Source: CAD feature listing. Evaluate the final solid. Frame: model axes, mm. A direction names the side the tool comes from. Round coordinates to 2 decimals unless told otherwise and drop trailing zeros. Loops run counter-clockwise (first coordinate to the right, second up) from the corner with the lowest first, then second, coordinate; pieces in that order, holes last. Notation, with made-up numbers: (50.25, 37) -> (100.25, 37) arc R33 ccw to (100.25, 73) -> close; hole circle Ø6 at (2, 25.5). An arc over 180 degrees is marked (long way). Put each result on its own line as item: value. Start each with the question number.
1. Contact query for flat-ended pins moving along their axis: pin 1 (6.5 mm diameter, centred on x = -65, y = 8, fed in from +Z); pin 2 (4.5 mm diameter, centred on y = 7, z = -56.5, fed in from +X); pin 3 (4 mm diameter, centred on x = -5.5, y = 10.5, fed in from -Z). Output: stop coordinate, or through.
2. Cut plane B-B (x = -39). Return the cut outline in (y, z), then the cut area to 3 significant figures.
3. Set-up query: faces 5 (the flat face through (49, 9, 56)), 6 (the flat face through (-13, 9, 56)), 7 (the flat face through (-17.1, 7.8, 54.25)). Return all of +Z, -Z, +X, -X, +Y, -Y with unobstructed straight access to the full face (end or side cutting, diameter ignored); none if empty.
4. Cut plane A-A (y = 10). State how many separate pieces and enclosed holes the cut face has, then the cut area to 3 significant figures.
5. Cut plane C-C (z = 31). Return the cut outline in (x, y), then the cut area to 3 significant figures.
6. Draft query along Z for faces 1 (the cylindrical face through (-6.06, 5.52, 1.04)), 2 (the flat face through (-1, 2, 62.5)), 3 (the flat face through (-3, 9, -56)), 4 (the flat face through (52.9, 7.8, 54.25)). Return one class per face: pulls with the +Z half, pulls with the -Z half, needs draft (parallel to the pull), parting line crosses it, or undercut.
7. Material intervals for L1, parallel to X at y = 4.5, z = 0.5; L2, parallel to X at y = 3.5, z = 0.5; L3, parallel to Y at x = -1, z = 3, sorted ascending.
```python
from build123d import *

# Parameters (mm, degrees)
SKETCH1_W                   = 154
SKETCH1_H                   = 125
BOSS_EXTRUDE1_DEPTH         = 4
CUT_EXTRUDE1_REACH          = 101.253
SKETCH3_R                   = 1.5
SKETCH15_R                  = 3
CUT_EXTRUDE7_DEPTH          = 2.5
CUT_EXTRUDE2_REACH          = 101.253
SKETCH4_R                   = 1.5
BOSS_EXTRUDE6_START         = 3
SKETCH17_R                  = 2.5
SKETCH17_R_2                = 1.5
BOSS_EXTRUDE6_DEPTH         = 3
LPATTERN1_COUNT             = 2
LPATTERN1_PITCH             = 58
LPATTERN2_COUNT             = 3
LPATTERN2_PITCH             = 49
LPATTERN2_COPY_1_REACH      = 101.253
LPATTERN2_COPY_1_SKETCH_R   = 1.5
LPATTERN2_COPY_2_REACH      = 101.253
LPATTERN2_COPY_2_SKETCH_R   = 1.5
LPATTERN2_START             = 3
LPATTERN2_COPY_3_SKETCH_R   = 2.5
LPATTERN2_COPY_3_SKETCH_R_2 = 1.5
LPATTERN2_COPY_3_DEPTH      = 3
LPATTERN2_COPY_4_SKETCH_R   = 2.5
LPATTERN2_COPY_4_SKETCH_R_2 = 1.5
LPATTERN2_COPY_4_DEPTH      = 3
LPATTERN3_COUNT             = 2
LPATTERN3_PITCH             = 75
LPATTERN3_COPY_1_REACH      = 101.253
LPATTERN3_COPY_1_SKETCH_R   = 1.5
LPATTERN3_START             = 3
LPATTERN3_COPY_2_SKETCH_R   = 2.5
LPATTERN3_COPY_2_SKETCH_R_2 = 1.5
LPATTERN3_COPY_2_DEPTH      = 3
SKETCH9_W                   = 8
SKETCH9_H                   = 4
BOSS_EXTRUDE4_DEPTH         = 10
CUT_EXTRUDE5_REACH          = 145.894
SKETCH10_R                  = 2
LPATTERN4_COUNT             = 2
LPATTERN4_PITCH             = 50
SKETCH12_W                  = 8
SKETCH12_H                  = 4
BOSS_EXTRUDE5_DEPTH         = 10
CUT_EXTRUDE6_REACH          = 144.588
SKETCH14_R                  = 2
LPATTERN5_COUNT             = 3
LPATTERN5_PITCH             = 60
LPATTERN6_COUNT             = 2
LPATTERN6_PITCH             = 120


with BuildPart() as part:
    # Sketch1 → Boss-Extrude1 (new body)
    with BuildSketch(Plane(origin=(0, 0, 0), x_dir=(1, 0, 0), z_dir=(0, 1, 0))):
        Rectangle(SKETCH1_W, SKETCH1_H)
    extrude(amount=BOSS_EXTRUDE1_DEPTH)

    # Sketch3 → Cut-Extrude1 (cut, up to next)
    with BuildSketch(Plane(origin=(0, 4, 0), x_dir=(1, 0, 0), z_dir=(0, 1, 0)), mode=Mode.PRIVATE) as cut_extrude1_sk1:
        with Locations(Location((-62.5, 37, 0), (0, 0, 270))):
            Circle(SKETCH3_R)
    cut_extrude1_tool1 = extrude(cut_extrude1_sk1.sketch, amount=-CUT_EXTRUDE1_REACH, mode=Mode.PRIVATE) & part.part
    cut_extrude1 = cut_extrude1_tool1.solids().sort_by_distance((-62.5, 4, -37))[0]
    add(cut_extrude1, mode=Mode.SUBTRACT)

    # Sketch15 → Cut-Extrude7 (cut)
    with BuildSketch(Plane.XZ):
        with Locations(Location((-62.5, -37, 0), (0, 0, 270))):
            Circle(SKETCH15_R)
    cut_extrude7 = extrude(amount=-CUT_EXTRUDE7_DEPTH, mode=Mode.SUBTRACT)

    # Mirror1: Cut-Extrude1, Cut-Extrude7 across plane
    add(cut_extrude1.mirror(Plane.XY), mode=Mode.SUBTRACT)
    add(cut_extrude7.mirror(Plane.XY), mode=Mode.SUBTRACT)

    # Sketch4 → Cut-Extrude2 (cut, up to next)
    with BuildSketch(Plane(origin=(0, 4, 0), x_dir=(1, 0, 0), z_dir=(0, 1, 0)), mode=Mode.PRIVATE) as cut_extrude2_sk1:
        with Locations(Location((49.5, -49.5, 0), (0, 0, 270))):
            Circle(SKETCH4_R)
    cut_extrude2_tool1 = extrude(cut_extrude2_sk1.sketch, amount=-CUT_EXTRUDE2_REACH, mode=Mode.PRIVATE) & part.part
    cut_extrude2 = cut_extrude2_tool1.solids().sort_by_distance((49.5, 4, 49.5))[0]
    add(cut_extrude2, mode=Mode.SUBTRACT)

    # Sketch17 → Boss-Extrude6 (add)
    with BuildSketch(Plane(origin=(0, 4, 0), x_dir=(1, 0, 0), z_dir=(0, 1, 0)).offset(BOSS_EXTRUDE6_START)):
        with Locations(Location((49.5, -49.5, 0), (0, 0, 90))):
            Circle(SKETCH17_R)
        with Locations(Location((49.5, -49.5, 0), (0, 0, 270))):
            Circle(SKETCH17_R_2, mode=Mode.SUBTRACT)
    boss_extrude6 = extrude(amount=-BOSS_EXTRUDE6_DEPTH)

    # LPattern1: Cut-Extrude2, Boss-Extrude6 ×2
    with Locations(*[(-i * LPATTERN1_PITCH, 0, 0) for i in range(1, LPATTERN1_COUNT)]):
        add(cut_extrude2, mode=Mode.SUBTRACT)
        add(boss_extrude6)

    # LPattern2: Cut-Extrude2, Boss-Extrude6 ×3
    with Locations(*[(0, 0, -i * LPATTERN2_PITCH) for i in range(1, LPATTERN2_COUNT)]):
        add(cut_extrude2, mode=Mode.SUBTRACT)
        add(boss_extrude6)

    # LPattern2 copy 1 sketch → LPattern2 copy 1 (cut, up to next)
    with BuildSketch(Plane(origin=(-58, 4, -49), x_dir=(1, 0, 0), z_dir=(0, 1, 0)), mode=Mode.PRIVATE) as lpattern2_copy_1_sk1:
        with Locations(Location((49.5, -49.5, 0), (0, 0, 270))):
            Circle(LPATTERN2_COPY_1_SKETCH_R)
    lpattern2_copy_1_tool1 = extrude(lpattern2_copy_1_sk1.sketch, amount=-LPATTERN2_COPY_1_REACH, mode=Mode.PRIVATE) & part.part
    add(lpattern2_copy_1_tool1.solids().sort_by_distance((-8.5, 4, 0.5))[0], mode=Mode.SUBTRACT)

    # LPattern2 copy 2 sketch → LPattern2 copy 2 (cut, up to next)
    with BuildSketch(Plane(origin=(-58, 4, -98), x_dir=(1, 0, 0), z_dir=(0, 1, 0)), mode=Mode.PRIVATE) as lpattern2_copy_2_sk1:
        with Locations(Location((49.5, -49.5, 0), (0, 0, 270))):
            Circle(LPATTERN2_COPY_2_SKETCH_R)
    lpattern2_copy_2_tool1 = extrude(lpattern2_copy_2_sk1.sketch, amount=-LPATTERN2_COPY_2_REACH, mode=Mode.PRIVATE) & part.part
    add(lpattern2_copy_2_tool1.solids().sort_by_distance((-8.5, 4, -48.5))[0], mode=Mode.SUBTRACT)

    # LPattern2 copy 3 sketch → LPattern2 copy 3 (add)
    with BuildSketch(Plane(origin=(-58, 4, -49), x_dir=(1, 0, 0), z_dir=(0, 1, 0)).offset(LPATTERN2_START)):
        with Locations(Location((49.5, -49.5, 0), (0, 0, 90))):
            Circle(LPATTERN2_COPY_3_SKETCH_R)
        with Locations(Location((49.5, -49.5, 0), (0, 0, 270))):
            Circle(LPATTERN2_COPY_3_SKETCH_R_2, mode=Mode.SUBTRACT)
    extrude(amount=-LPATTERN2_COPY_3_DEPTH)

    # LPattern2 copy 4 sketch → LPattern2 copy 4 (add)
    with BuildSketch(Plane(origin=(-58, 4, -98), x_dir=(1, 0, 0), z_dir=(0, 1, 0)).offset(LPATTERN2_START)):
        with Locations(Location((49.5, -49.5, 0), (0, 0, 90))):
            Circle(LPATTERN2_COPY_4_SKETCH_R)
        with Locations(Location((49.5, -49.5, 0), (0, 0, 270))):
            Circle(LPATTERN2_COPY_4_SKETCH_R_2, mode=Mode.SUBTRACT)
    extrude(amount=-LPATTERN2_COPY_4_DEPTH)

    # LPattern3: Cut-Extrude2, Boss-Extrude6 ×2
    with Locations(*[(0, 0, -i * LPATTERN3_PITCH) for i in range(1, LPATTERN3_COUNT)]):
        add(cut_extrude2, mode=Mode.SUBTRACT)
        add(boss_extrude6)

    # LPattern3 copy 1 sketch → LPattern3 copy 1 (cut, up to next)
    with BuildSketch(Plane(origin=(-58, 4, -75), x_dir=(1, 0, 0), z_dir=(0, 1, 0)), mode=Mode.PRIVATE) as lpattern3_copy_1_sk1:
        with Locations(Location((49.5, -49.5, 0), (0, 0, 270))):
            Circle(LPATTERN3_COPY_1_SKETCH_R)
    lpattern3_copy_1_tool1 = extrude(lpattern3_copy_1_sk1.sketch, amount=-LPATTERN3_COPY_1_REACH, mode=Mode.PRIVATE) & part.part
    add(lpattern3_copy_1_tool1.solids().sort_by_distance((-8.5, 4, -25.5))[0], mode=Mode.SUBTRACT)

    # LPattern3 copy 2 sketch → LPattern3 copy 2 (add)
    with BuildSketch(Plane(origin=(-58, 4, -75), x_dir=(1, 0, 0), z_dir=(0, 1, 0)).offset(LPATTERN3_START)):
        with Locations(Location((49.5, -49.5, 0), (0, 0, 90))):
            Circle(LPATTERN3_COPY_2_SKETCH_R)
        with Locations(Location((49.5, -49.5, 0), (0, 0, 270))):
            Circle(LPATTERN3_COPY_2_SKETCH_R_2, mode=Mode.SUBTRACT)
    extrude(amount=-LPATTERN3_COPY_2_DEPTH)

    # Sketch9 → Boss-Extrude4 (add)
    with BuildSketch(Plane(origin=(0, 4, 0), x_dir=(1, 0, 0), z_dir=(0, 1, 0))):
        with Locations((-67, -56.25)):
            Rectangle(SKETCH9_W, SKETCH9_H)
    boss_extrude4 = extrude(amount=BOSS_EXTRUDE4_DEPTH)

    # Sketch10 → Cut-Extrude5 (cut, up to next)
    with BuildSketch(Plane.XY.offset(58.25), mode=Mode.PRIVATE) as cut_extrude5_sk1:
        with Locations((-67, 10)):
            Circle(SKETCH10_R)
    cut_extrude5_tool1 = extrude(cut_extrude5_sk1.sketch, amount=-CUT_EXTRUDE5_REACH, mode=Mode.PRIVATE) & part.part
    cut_extrude5 = cut_extrude5_tool1.solids().sort_by_distance((-67, 10, 58.25))[0]
    add(cut_extrude5, mode=Mode.SUBTRACT)

    # LPattern4: Boss-Extrude4, Cut-Extrude5 ×2
    with Locations(*[(i * LPATTERN4_PITCH, 0, 0) for i in range(1, LPATTERN4_COUNT)]):
        add(boss_extrude4)
        add(cut_extrude5, mode=Mode.SUBTRACT)

    # Sketch12 → Boss-Extrude5 (add)
    with BuildSketch(Plane(origin=(-3.289149479, 4, -108.840697075), x_dir=(1, 0, 0), z_dir=(0, 1, 0))):
        with Locations((-63.710850521, -52.340697075)):
            Rectangle(SKETCH12_W, SKETCH12_H)
    boss_extrude5 = extrude(amount=BOSS_EXTRUDE5_DEPTH)

    # Sketch14 → Cut-Extrude6 (cut, up to next)
    with BuildSketch(Plane(origin=(-3.289149479, 0, -54.5), x_dir=(1, 0, 0), z_dir=(0, 0, 1)), mode=Mode.PRIVATE) as cut_extrude6_sk1:
        with Locations((-63.710850521, 10)):
            Circle(SKETCH14_R)
    cut_extrude6_tool1 = extrude(cut_extrude6_sk1.sketch, amount=-CUT_EXTRUDE6_REACH, mode=Mode.PRIVATE) & part.part
    cut_extrude6 = cut_extrude6_tool1.solids().sort_by_distance((-67, 10, -54.5))[0]
    add(cut_extrude6, mode=Mode.SUBTRACT)

    # LPattern5: Boss-Extrude5, Cut-Extrude6 ×3
    with Locations(*[(i * LPATTERN5_PITCH, 0, 0) for i in range(1, LPATTERN5_COUNT)]):
        add(boss_extrude5)
        add(cut_extrude6, mode=Mode.SUBTRACT)

    # LPattern6: Boss-Extrude4, Cut-Extrude5 ×2
    with Locations(*[(i * LPATTERN6_PITCH, 0, 0) for i in range(1, LPATTERN6_COUNT)]):
        add(boss_extrude4)
        add(cut_extrude5, mode=Mode.SUBTRACT)


solid = part.part
```
Solution:
1. pin 1: stops at z = 58.25
1. pin 2: stops at x = 57
1. pin 3: stops at z = -58.5
2. outline: (0, -62.5) -> (4, -62.5) -> (4, 62.5) -> (0, 62.5) -> close
2. area: 500 mm^2
3. face 5: +Z, +Y
3. face 6: +Z, -Z, +Y
3. face 7: -Z, +X, -X, +Y
4. separate pieces: 12
4. enclosed holes: 0
4. area: 96.0 mm^2
5. outline: (-77, 0) -> (77, 0) -> (77, 4) -> (-77, 4) -> close
5. area: 616 mm^2
6. face 1: undercut
6. face 2: pulls with the +Z half
6. face 3: needs draft
6. face 4: undercut
7. L1: x = -11 to -10, -7 to -6, 47 to 48, 51 to 52
7. L2: x = -77 to -10, -7 to 48, 51 to 77
7. L3: y = 0 to 4
